Read the model definition and answer for the solid it produces. Units are mm, in the model's axes. Give positions to 0.01 mm unless a question says otherwise; leave off trailing zeros. Put each result on its own line as item: value.
from build123d import *

# Parameters (mm, degrees)
SKETCH2_W            = 215.1
SKETCH2_H            = 34.9
BOSS_EXTRUDE1_DEPTH  = 2
M3_CLEARANCE_HOLE1_D = 3.4
CUT_EXTRUDE1_REACH   = 136.214
SKETCH7_R            = 2.5


with BuildPart() as part:
    # Sketch2 → Boss-Extrude1 (new body)
    with BuildSketch(Plane(origin=(0, 0, 0), x_dir=(1, 0, 0), z_dir=(0, 1, 0))):
        with Locations((-22.149288499, -17.010354253)):
            Rectangle(SKETCH2_W, SKETCH2_H)
    extrude(amount=BOSS_EXTRUDE1_DEPTH)

    # M3 Clearance Hole1 (through all)
    with Locations(Plane(origin=(0, 2, 0), x_dir=(1, 0, 0), z_dir=(0, 1, 0))):
        with Locations((-122.199288499, -2.060354253), (-122.199288499, -31.960354253), (77.900711501, -2.060354253), (77.900711501, -31.960354253)):
            Hole(M3_CLEARANCE_HOLE1_D / 2)

    # Sketch7 → Cut-Extrude1 (cut, up to next)
    with BuildSketch(Plane.XZ, mode=Mode.PRIVATE) as cut_extrude1_sk1:
        with Locations(Location((-108.189288499, 19.460354253, 0), (0, 0, 270))):
            Circle(SKETCH7_R)
    cut_extrude1_tool1 = extrude(cut_extrude1_sk1.sketch, amount=-CUT_EXTRUDE1_REACH, mode=Mode.PRIVATE) & part.part
    # Sketch7 → Cut-Extrude1 (cut, up to next)
    with BuildSketch(Plane.XZ, mode=Mode.PRIVATE) as cut_extrude1_sk2:
        with Locations(Location((-65.169288499, 19.460354253, 0), (0, 0, 270))):
            Circle(SKETCH7_R)
    cut_extrude1_tool2 = extrude(cut_extrude1_sk2.sketch, amount=-CUT_EXTRUDE1_REACH, mode=Mode.PRIVATE) & part.part
    # Sketch7 → Cut-Extrude1 (cut, up to next)
    with BuildSketch(Plane.XZ, mode=Mode.PRIVATE) as cut_extrude1_sk3:
        with Locations(Location((-22.149288499, 19.460354253, 0), (0, 0, 270))):
            Circle(SKETCH7_R)
    cut_extrude1_tool3 = extrude(cut_extrude1_sk3.sketch, amount=-CUT_EXTRUDE1_REACH, mode=Mode.PRIVATE) & part.part
    # Sketch7 → Cut-Extrude1 (cut, up to next)
    with BuildSketch(Plane.XZ, mode=Mode.PRIVATE) as cut_extrude1_sk4:
        with Locations(Location((20.870711501, 19.460354253, 0), (0, 0, 270))):
            Circle(SKETCH7_R)
    cut_extrude1_tool4 = extrude(cut_extrude1_sk4.sketch, amount=-CUT_EXTRUDE1_REACH, mode=Mode.PRIVATE) & part.part
    # Sketch7 → Cut-Extrude1 (cut, up to next)
    with BuildSketch(Plane.XZ, mode=Mode.PRIVATE) as cut_extrude1_sk5:
        with Locations(Location((63.890711501, 19.460354253, 0), (0, 0, 270))):
            Circle(SKETCH7_R)
    cut_extrude1_tool5 = extrude(cut_extrude1_sk5.sketch, amount=-CUT_EXTRUDE1_REACH, mode=Mode.PRIVATE) & part.part
    add(cut_extrude1_tool1.solids().sort_by_distance((-108.189288, 0, 19.460354))[0], mode=Mode.SUBTRACT)
    add(cut_extrude1_tool2.solids().sort_by_distance((-65.169288, 0, 19.460354))[0], mode=Mode.SUBTRACT)
    add(cut_extrude1_tool3.solids().sort_by_distance((-22.149288, 0, 19.460354))[0], mode=Mode.SUBTRACT)
    add(cut_extrude1_tool4.solids().sort_by_distance((20.870712, 0, 19.460354))[0], mode=Mode.SUBTRACT)
    add(cut_extrude1_tool5.solids().sort_by_distance((63.890712, 0, 19.460354))[0], mode=Mode.SUBTRACT)


solid = part.part
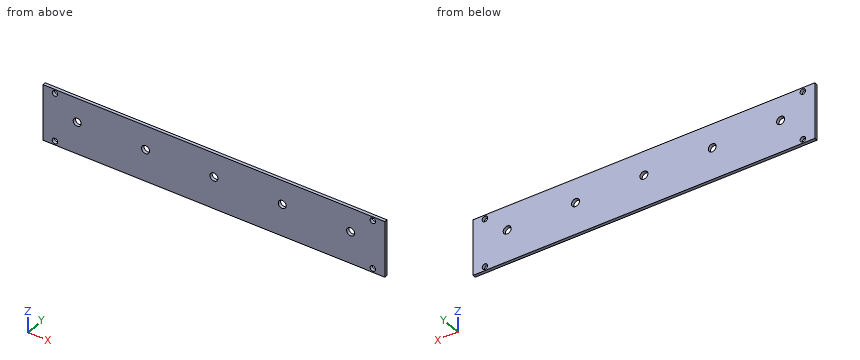
(1) Given pin 1 Ø6 at (x, z) = (-108.19, 19.46) entering from +Y; pin 2 Ø3 at (x, z) = (-122.2, 31.96) entering from +Y, each flat-ended and moving along its own axis, determine where each tip first touches the part or whether it passes through.
Result:
pin 1: stops at y = 2
pin 2: passes through
(2) Straight lines are drawn through the part: line 1 along X through (y, z) = (0.15, 32); line 2 along X through (y, z) = (0.95, 19.5); line 3 along X through (y, z) = (1.5, 19). For each, find the intervals that lie inside material, in ascending order. Write a range as from..to.
Result:
line 1: x = -129.7..-123.9, -120.5..76.2, 79.6..85.4
line 2: x = -129.7..-110.69, -105.69..-67.67, -62.67..-24.65, -19.65..18.37, 23.37..61.39, 66.39..85.4
line 3: x = -129.7..-110.65, -105.73..-67.63, -62.71..-24.61, -19.69..18.41, 23.33..61.43, 66.35..85.4
(3) Section A-A on y = 0.4 is taken. Give the number of separate pieces and of enclosed holes in the cut face, and give its area (3 significant figures).
Result:
separate pieces: 1
enclosed holes: 9
area: 7,370 mm²
